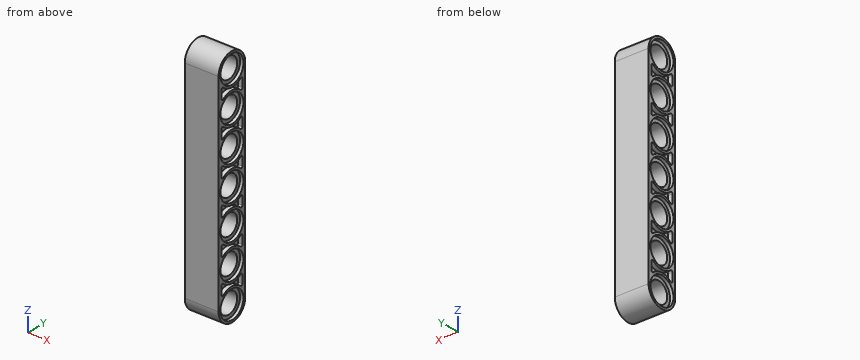
```python
from build123d import *

# Parameters (mm, degrees)
SKETCH1_R           = 2.4
BOSS_EXTRUDE1_DEPTH = 8
SKETCH2_R           = 3.2
CUT_EXTRUDE1_DEPTH  = 0.8
CUT_EXTRUDE2_START  = -1
CUT_EXTRUDE2_DEPTH  = 1


with BuildPart() as part:
    # Sketch1 → Boss-Extrude1 (new body)
    with BuildSketch(Plane(origin=(0, 0, 0), x_dir=(0, 0, -1), z_dir=(1, 0, 0))):
        with BuildLine():
            Line((-10.64973545, 3.7), (37.35026455, 3.7))
            ThreePointArc((37.35026455, 3.7), (41.05026455, 0), (37.35026455, -3.7))
            Line((37.35026455, -3.7), (-10.64973545, -3.7))
            ThreePointArc((-10.64973545, -3.7), (-14.34973545, 0), (-10.64973545, 3.7))
        make_face()
        with Locations((-10.64973545, 0)):
            Circle(SKETCH1_R, mode=Mode.SUBTRACT)
        with Locations((-2.64973545, 0)):
            Circle(SKETCH1_R, mode=Mode.SUBTRACT)
        with Locations((5.35026455, 0)):
            Circle(SKETCH1_R, mode=Mode.SUBTRACT)
        with Locations((13.35026455, 0)):
            Circle(SKETCH1_R, mode=Mode.SUBTRACT)
        with Locations((21.35026455, 0)):
            Circle(SKETCH1_R, mode=Mode.SUBTRACT)
        with Locations((29.35026455, 0)):
            Circle(SKETCH1_R, mode=Mode.SUBTRACT)
        with Locations((37.35026455, 0)):
            Circle(SKETCH1_R, mode=Mode.SUBTRACT)
    extrude(amount=BOSS_EXTRUDE1_DEPTH)

    # Sketch2 → Cut-Extrude1 (cut)
    with BuildSketch(Plane(origin=(8, 0, 0), x_dir=(0, 0, -1), z_dir=(1, 0, 0))):
        with Locations((-10.64973545, 0)):
            Circle(SKETCH2_R)
        with Locations((-2.64973545, 0)):
            Circle(SKETCH2_R)
        with Locations((5.35026455, 0)):
            Circle(SKETCH2_R)
        with Locations((13.35026455, 0)):
            Circle(SKETCH2_R)
        with Locations((21.35026455, 0)):
            Circle(SKETCH2_R)
        with Locations((29.35026455, 0)):
            Circle(SKETCH2_R)
        with Locations((37.35026455, 0)):
            Circle(SKETCH2_R)
    cut_extrude1 = extrude(amount=-CUT_EXTRUDE1_DEPTH, mode=Mode.SUBTRACT)

    # Sketch3 → Cut-Extrude2 (cut)
    with BuildSketch(Plane(origin=(8, 0, 0), x_dir=(0, 0, -1), z_dir=(1, 0, 0)).offset(CUT_EXTRUDE2_START)):
        with BuildLine():
            Line((-7.609998619, 2.9), (-5.68947228, 2.9))
            ThreePointArc((-5.68947228, 2.9), (-5.416983749, 2.725499004), (-5.461492018, 2.405))
            ThreePointArc((-5.461492018, 2.405), (-6.34973545, 0), (-5.461492018, -2.405))
            ThreePointArc((-5.461492018, -2.405), (-5.416983749, -2.725499004), (-5.68947228, -2.9))
            Line((-5.68947228, -2.9), (-7.609998619, -2.9))
            ThreePointArc((-7.609998619, -2.9), (-7.882487151, -2.725499004), (-7.837978881, -2.405))
            ThreePointArc((-7.837978881, -2.405), (-6.94973545, 0), (-7.837978881, 2.405))
            ThreePointArc((-7.837978881, 2.405), (-7.882487151, 2.725499004), (-7.609998619, 2.9))
        make_face()
        with BuildLine():
            Line((0.390001381, 2.9), (2.31052772, 2.9))
            ThreePointArc((2.31052772, 2.9), (2.583016251, 2.725499004), (2.538507982, 2.405))
            ThreePointArc((2.538507982, 2.405), (1.65026455, 0), (2.538507982, -2.405))
            ThreePointArc((2.538507982, -2.405), (2.583016251, -2.725499004), (2.31052772, -2.9))
            Line((2.31052772, -2.9), (0.390001381, -2.9))
            ThreePointArc((0.390001381, -2.9), (0.117512849, -2.725499004), (0.162021119, -2.405))
            ThreePointArc((0.162021119, -2.405), (1.05026455, 0), (0.162021119, 2.405))
            ThreePointArc((0.162021119, 2.405), (0.117512849, 2.725499004), (0.390001381, 2.9))
        make_face()
        with BuildLine():
            Line((8.390001381, 2.9), (10.31052772, 2.9))
            ThreePointArc((10.31052772, 2.9), (10.583016251, 2.725499004), (10.538507982, 2.405))
            ThreePointArc((10.538507982, 2.405), (9.65026455, 0), (10.538507982, -2.405))
            ThreePointArc((10.538507982, -2.405), (10.583016251, -2.725499004), (10.31052772, -2.9))
            Line((10.31052772, -2.9), (8.390001381, -2.9))
            ThreePointArc((8.390001381, -2.9), (8.117512849, -2.725499004), (8.162021119, -2.405))
            ThreePointArc((8.162021119, -2.405), (9.05026455, 0), (8.162021119, 2.405))
            ThreePointArc((8.162021119, 2.405), (8.117512849, 2.725499004), (8.390001381, 2.9))
        make_face()
        with BuildLine():
            Line((16.390001381, 2.9), (18.31052772, 2.9))
            ThreePointArc((18.31052772, 2.9), (18.583016251, 2.725499004), (18.538507982, 2.405))
            ThreePointArc((18.538507982, 2.405), (17.65026455, 0), (18.538507982, -2.405))
            ThreePointArc((18.538507982, -2.405), (18.583016251, -2.725499004), (18.31052772, -2.9))
            Line((18.31052772, -2.9), (16.390001381, -2.9))
            ThreePointArc((16.390001381, -2.9), (16.117512849, -2.725499004), (16.162021119, -2.405))
            ThreePointArc((16.162021119, -2.405), (17.05026455, 0), (16.162021119, 2.405))
            ThreePointArc((16.162021119, 2.405), (16.117512849, 2.725499004), (16.390001381, 2.9))
        make_face()
        with BuildLine():
            Line((24.390001381, 2.9), (26.31052772, 2.9))
            ThreePointArc((26.31052772, 2.9), (26.583016251, 2.725499004), (26.538507982, 2.405))
            ThreePointArc((26.538507982, 2.405), (25.65026455, 0), (26.538507982, -2.405))
            ThreePointArc((26.538507982, -2.405), (26.583016251, -2.725499004), (26.31052772, -2.9))
            Line((26.31052772, -2.9), (24.390001381, -2.9))
            ThreePointArc((24.390001381, -2.9), (24.117512849, -2.725499004), (24.162021119, -2.405))
            ThreePointArc((24.162021119, -2.405), (25.05026455, 0), (24.162021119, 2.405))
            ThreePointArc((24.162021119, 2.405), (24.117512849, 2.725499004), (24.390001381, 2.9))
        make_face()
        with BuildLine():
            Line((32.390001381, 2.9), (34.31052772, 2.9))
            ThreePointArc((34.31052772, 2.9), (34.583016251, 2.725499004), (34.538507982, 2.405))
            ThreePointArc((34.538507982, 2.405), (33.65026455, 0), (34.538507982, -2.405))
            ThreePointArc((34.538507982, -2.405), (34.583016251, -2.725499004), (34.31052772, -2.9))
            Line((34.31052772, -2.9), (32.390001381, -2.9))
            ThreePointArc((32.390001381, -2.9), (32.117512849, -2.725499004), (32.162021119, -2.405))
            ThreePointArc((32.162021119, -2.405), (33.05026455, 0), (32.162021119, 2.405))
            ThreePointArc((32.162021119, 2.405), (32.117512849, 2.725499004), (32.390001381, 2.9))
        make_face()
    cut_extrude2 = extrude(amount=CUT_EXTRUDE2_DEPTH, mode=Mode.SUBTRACT)

    # Mirror1: Cut-Extrude1, Cut-Extrude2 across plane
    add(cut_extrude1.mirror(Plane(origin=(4, 0, 0), x_dir=(0, 0, 1), z_dir=(1, 0, 0))), mode=Mode.SUBTRACT)
    add(cut_extrude2.mirror(Plane(origin=(4, 0, 0), x_dir=(0, 0, 1), z_dir=(1, 0, 0))), mode=Mode.SUBTRACT)


solid = part.part
```
Input: part model. Units: mm. Frame: model coordinates. Coordinates: 2 decimals unless noted, no trailing zeros. Write each loop counter-clockwise with the first axis right and the second up, starting at its lowest first coordinate (ties: lowest second). Pieces come first, ordered by that corner, then holes. Notation, with made-up numbers: (20.5, 41.5) -> (24.5, 41.5) arc R29 cw to (24.5, 71.5) -> close; hole circle Ø5 at (33, 12.5). An arc over 180 degrees is marked (long way). Answer as a JSON object with one key per item and string values.
1. Section B-B on x = 2. Return the cut outline in (y, z).
Result set:
{"outline": "(-3.7, -37.35) arc R3.7 ccw to (3.7, -37.35) -> (3.7, 10.65) arc R3.7 ccw to (-3.7, 10.65) -> close; hole circle Ø4.8 at (0, -37.35); hole circle Ø4.8 at (0, -29.35); hole circle Ø4.8 at (0, -21.35); hole circle Ø4.8 at (0, -13.35); hole circle Ø4.8 at (0, -5.35); hole circle Ø4.8 at (0, 2.65); hole circle Ø4.8 at (0, 10.65)"}
2. Section D-D on z = 2.5. Return the cut outline in (x, y).
Result set:
{"outline": "(0, -3.7) -> (8, -3.7) -> (8, -3.2) -> (7.2, -3.2) -> (7.2, -2.4) -> (0.8, -2.4) -> (0.8, -3.2) -> (0, -3.2) -> close; (0, 3.2) -> (0.8, 3.2) -> (0.8, 2.4) -> (7.2, 2.4) -> (7.2, 3.2) -> (8, 3.2) -> (8, 3.7) -> (0, 3.7) -> close"}
3. Section C-C on y = 0. Count the separate pieces of the cut face and the enclosed holes in it, then the cut area to 3 significant figures.
Result set:
{"separate pieces": "8", "enclosed holes": "0", "area": "149 mm2"}
4. Material intervals for line 1 (Y direction, x = 4, z = 2.5); line 2 (Y direction, x = 6, z = -28); line 3 (X direction, y = -2.25, z = 12), sorted ascending. Write a range as from..to.
Result set:
{"line 1": "y = -3.7..-2.4, 2.4..3.7", "line 2": "y = -3.7..-1.98, 1.98..3.7", "line 3": "x = 0.8..7.2"}
5. First-contact query: P1, Ø1, axis at y = 1.5, z = -5, coming from the +X side; P2, Ø3, axis at y = -1, z = 1, coming from the -X side. Flat tips, straight axial feed; report the tip coordinate or a pass-through.
Result set:
{"P1": "passes through", "P2": "stops at x = 0"}
6. Section A-A on z = -22.5. Return the cut outline in (x, y), then the cut area to 3 significant figures.
Result set:
{"outline": "(0, -3.7) -> (8, -3.7) -> (8, -2.99) -> (7.2, -2.99) -> (7.2, -2.11) -> (0.8, -2.11) -> (0.8, -2.99) -> (0, -2.99) -> close; (0, 2.99) -> (0.8, 2.99) -> (0.8, 2.11) -> (7.2, 2.11) -> (7.2, 2.99) -> (8, 2.99) -> (8, 3.7) -> (0, 3.7) -> close", "area": "22.7 mm2"}
